```python
from build123d import *

# Parameters (mm, degrees)
BOSS_EXTRUDE1_DEPTH     = 2
SKETCH5_R               = 30.25
BOSS_EXTRUDE2_DEPTH     = 3
SKETCH6_R               = 7.25
SKETCH6_R_2             = 5.75
BOSS_EXTRUDE3_DEPTH     = 6
SKETCH7_R               = 1
CUT_EXTRUDE1_DEPTH      = 10
CUT_EXTRUDE1_DEPTH_BACK = 3


with BuildPart() as part:
    # Sketch3 → Boss-Extrude1 (new body)
    with BuildSketch(Plane.XY):
        with BuildLine():
            Line((22.900234193, 23.5), (-22.900234193, 23.5))
            ThreePointArc((-22.900234193, 23.5), (-76, 0), (-22.900234193, -23.5))
            Line((-22.900234193, -23.5), (22.900234193, -23.5))
            ThreePointArc((22.900234193, -23.5), (76, 0), (22.900234193, 23.5))
        make_face()
    extrude(amount=BOSS_EXTRUDE1_DEPTH)

    # Sketch5 → Boss-Extrude2 (add)
    with BuildSketch(Plane.XY.offset(2)):
        with BuildLine():
            Line((22.900234193, 23.5), (-22.900234193, 23.5))
            ThreePointArc((-22.900234193, 23.5), (-76, 0), (-22.900234193, -23.5))
            Line((-22.900234193, -23.5), (22.900234193, -23.5))
            ThreePointArc((22.900234193, -23.5), (76, 0), (22.900234193, 23.5))
        make_face()
        with Locations((-44.25, 0)):
            Circle(SKETCH5_R, mode=Mode.SUBTRACT)
        with Locations((44.25, 0)):
            Circle(SKETCH5_R, mode=Mode.SUBTRACT)
        with BuildLine():
            Line((-21.357588594, 22), (21.357588594, 22))
            ThreePointArc((21.357588594, 22), (12.5, 0), (21.357588594, -22))
            Line((21.357588594, -22), (-21.357588594, -22))
            ThreePointArc((-21.357588594, -22), (-12.5, 0), (-21.357588594, 22))
        make_face(mode=Mode.SUBTRACT)
    extrude(amount=BOSS_EXTRUDE2_DEPTH)

    # Sketch6 → Boss-Extrude3 (add)
    with BuildSketch(Plane.XY.offset(2)):
        with Locations((-44.25, 0)):
            Circle(SKETCH6_R)
        with Locations((-44.25, 0)):
            Circle(SKETCH6_R_2, mode=Mode.SUBTRACT)
        with Locations((44.447055655, -0.28653356)):
            Circle(SKETCH6_R)
        with Locations((44.447055655, -0.28653356)):
            Circle(SKETCH6_R_2, mode=Mode.SUBTRACT)
    extrude(amount=BOSS_EXTRUDE3_DEPTH)

    # Sketch7 → Cut-Extrude1 (cut, two sides)
    with BuildSketch(Plane.XY.offset(2)) as cut_extrude1_sk:
        with Locations((0, 18.5)):
            Circle(SKETCH7_R)
        with Locations((0, -18.5)):
            Circle(SKETCH7_R)
    extrude(amount=CUT_EXTRUDE1_DEPTH, mode=Mode.SUBTRACT)
    extrude(cut_extrude1_sk.sketch, amount=-CUT_EXTRUDE1_DEPTH_BACK, mode=Mode.SUBTRACT)


solid = part.part
```
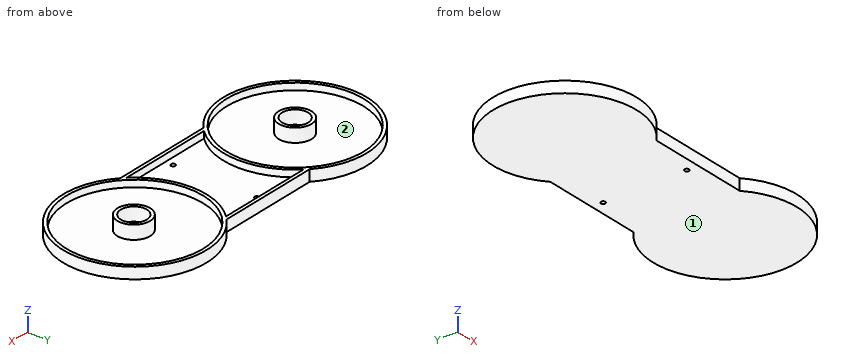
Here's how the part is built. I have some questions about the finished solid (model axes, mm). Face numbers are marked on the shaded views. Round coordinates to 2 decimals unless told otherwise and drop trailing zeros. Order: outer loops, then holes, each group sorted by start corner. A loop starts at its lowest first (then second) coordinate and runs counter-clockwise, first axis right, second up. Notation, with made-up numbers: M 84,72.5 L 141,72.5 A27 cw 141,90.5 Z; hole C 24.25,46.25 d9. An arc over 180 degrees is marked long. One line per question, with ' | ' between items.
1) I want a section at C-C, the plane x = 31.5. Write out the boundary of the cut face in (y, z), then the cut area to 3 significant figures.
Working result:
outline: M -29.08,0 L 29.08,0 L 29.08,5 L 27.43,5 L 27.43,2 L -27.43,2 L -27.43,5 L -29.08,5 Z | area: 126 mm²
2) I need wall thicknesses on line 1 along Y through (x, z) = (0, 1.1); line 2 along Y through (x, z) = (-44.25, 3.05); line 3 along X through (y, z) = (-17, 2.25). Which ranges of each line are inside material? Lowest first, please.
Working result:
line 1: -23.5 to -19.5, -17.5 to 17.5, 19.5 to 23.5 | line 2: -31.75 to -30.25, -7.25 to -5.75, 5.75 to 7.25, 30.25 to 31.75 | line 3: -71.07 to -69.27, -19.23 to -17.43, 17.43 to 19.23, 69.27 to 71.07
3) I want a section at A-A, the plane x = -44.25. Write out the boundary of the cut face in (y, z), then the cut area to 3 significant figures.
Working result:
outline: M -31.75,0 L 31.75,0 L 31.75,5 L 30.25,5 L 30.25,2 L 7.25,2 L 7.25,8 L 5.75,8 L 5.75,2 L -5.75,2 L -5.75,8 L -7.25,8 L -7.25,2 L -30.25,2 L -30.25,5 L -31.75,5 Z | area: 154 mm²
4) I want a section at B-B, the plane y = 16. Write out the boundary of the cut face in (x, z).
Working result:
outline: M -71.67,0 L 71.67,0 L 71.67,5 L 69.92,5 L 69.92,2 L 18.58,2 L 18.58,5 L 16.83,5 L 16.83,2 L -16.83,2 L -16.83,5 L -18.58,5 L -18.58,2 L -69.92,2 L -69.92,5 L -71.67,5 Z
5) For pin 1 Ø21.5 at (x, y) = (9, 5) entering from +Z; pin 2 Ø4 at (x, z) = (-13.5, 6) entering from +Y; pin 3 Ø1 at (x, z) = (-37.5, 2) entering from +Y, each with a flat end and sliding along its axis, tell me the tip position at first contact or that it passes through.
Working result:
pin 1: z = 5 | pin 2: y = 23.5 | pin 3: y = 31.13
6) I want a section at D-D, the plane x = -65.5. Write out the boundary of the cut face in (y, z).
Working result:
outline: M -23.59,0 L 23.59,0 L 23.59,5 L 21.53,5 L 21.53,2 L -21.53,2 L -21.53,5 L -23.59,5 Z
7) If we mould it in two halves opening along X, with no side actions, what happens to the marked faces 1 and 2? For each: +X half, -X half, draft (parallel to the pull), parting line (faces both ways), or undercut.
Working result:
face 1: draft | face 2: undercut
